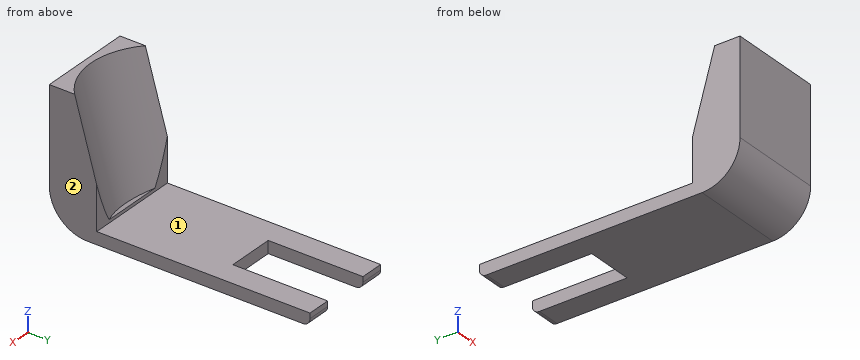
```python
from build123d import *

# Parameters (mm, degrees)
BOX001_W            = 10
BOX001_H            = 25
BOX001_DEPTH        = 10
BOX_W               = 20
BOX_H               = 45
BOX_DEPTH           = 2.6
CYLINDER_R          = 15
CYLINDER_DEPTH      = 27
CYLINDER_ROLL_ANGLE = 15.99999
BOX002_W            = 20
BOX002_H            = 10
BOX002_DEPTH        = 28
FILLET_R            = 8
FILLET001_R         = 1.5


with BuildPart() as box02:
    # Box001 → Box001 (new body)
    with BuildSketch(Plane(origin=(5, 25, -3), x_dir=(1, 0, 0), z_dir=(0, 0, 1))):
        with Locations((5, 12.5)):
            Rectangle(BOX001_W, BOX001_H)
    extrude(amount=BOX001_DEPTH)


with BuildPart() as obj1:
    # Box → Box (new body)
    with BuildSketch(Plane.XY):
        with Locations((10, 22.5)):
            Rectangle(BOX_W, BOX_H)
    extrude(amount=BOX_DEPTH)

    # Cut: cut Box02
    add(box02.part, mode=Mode.SUBTRACT)


with BuildPart() as cylinder:
    # Cylinder → Cylinder (new body)
    with BuildSketch(Plane.XY):
        Circle(CYLINDER_R)
    extrude(amount=CYLINDER_DEPTH)


with BuildPart() as cylinder_1:
    # Cylinder roll: moved
    add(cylinder.part.rotate(Axis((0, 0, 0), (1, 0, 0)), CYLINDER_ROLL_ANGLE))


with BuildPart() as cylinder_2:
    # Cylinder placement: moved
    add(cylinder_1.part.moved(Location((10, 13, 7))))


with BuildPart() as fillet001:
    # Box002 → Box002 (new body)
    with BuildSketch(Plane(origin=(0, -10, 0), x_dir=(1, 0, 0), z_dir=(0, 0, 1))):
        with Locations((10, 5)):
            Rectangle(BOX002_W, BOX002_H)
    extrude(amount=BOX002_DEPTH)

    # Fillet
    fillet_edges = [fillet001.edges().sort_by_distance(p)[0] for p in [
        (10, -10, 0),
    ]]
    fillet(fillet_edges, radius=FILLET_R)

    # Cut001: cut Cylinder
    add(cylinder_2.part, mode=Mode.SUBTRACT)

    # Fusion: union obj1
    add(obj1.part)

    # Fillet001
    fillet001_edges = [fillet001.edges().sort_by_distance(p)[0] for p in [
        (17.5, 45, 0),
        (2.5, 45, 0),
    ]]
    fillet(fillet001_edges, radius=FILLET001_R)


solid = fillet001.part
```
For this review, take the finished solid that the model builds, in its own axes (mm). Face numbers are marked on the shaded views. A direction names the side the tool comes from. Coordinates: 2 decimals unless noted, no trailing zeros. Order: outer loops, then holes, each group sorted by start corner. A loop starts at its lowest first (then second) coordinate and runs counter-clockwise, first axis right, second up. Notation, with made-up numbers: (41.25, 71.5) -> (46.25, 71.5) arc R14 ccw to (46.25, 88.5) -> close; hole circle Ø7 at (86.25, 3.5). An arc over 180 degrees is marked (long way). Use CSV: the item, a comma, the result in double quotes. Start each with the question number.
Item 1: We need section C-C, the plane y = 7.5. Give the boundary of the cut face in (x, z), then the cut area to 3 significant figures.
Item 2: Insertion check: pin 1 (3 mm diameter, centred on x = 6, z = 6.5, fed in from +Y); pin 2 (0.8 mm diameter, centred on x = 10.5, z = 1, fed in from +Y); pin 3 (5 mm diameter, centred on x = 18, z = 11.5, fed in from +Y). Each pin has a flat end and moves straight along its axis. Give the tip position at first contact, or say it passes through.
Item 3: We need section A-A, the plane y = 39. Give the boundary of the cut face in (x, z), then the cut area to 3 significant figures.
Item 4: We need section D-D, the plane x = 6.25. Give the boundary of the cut face in (y, z), then the cut area to 3 significant figures.
Item 5: Wall thickness on probe 1 along Z at (x, y) = (5.5, 9); probe 2 along Y at (x, z) = (18.25, 6); probe 3 along Y at (x, z) = (16.5, 19.75): over which ranges is each line inside the solid? List them lowest first.
Item 6: For the marked faces 1 and 2, list the 3-axis set-ups (+Z, -Z, +X, -X, +Y, -Y) from which the entire face can be reached by the end or side of a thin tool; tool diameter is ignored.
Item 7: We need section B-B, the plane x = 2. Give the boundary of the cut face in (y, z), then the cut area to 3 significant figures.
Derived:
1,outline,"(0, 0) -> (20, 0) -> (20, 2.6) -> (0, 2.6) -> close"
1,area,"52.0 mm^2"
2,pin 1,"stops at y = -1.24"
2,pin 2,"stops at y = 25"
2,pin 3,"stops at y = 0"
3,outline,"(0, 0) -> (5, 0) -> (5, 2.6) -> (0, 2.6) -> close; (15, 0) -> (20, 0) -> (20, 2.6) -> (15, 2.6) -> close"
3,area,"26.0 mm^2"
4,outline,"(-10, 8) arc R8 ccw to (-2, 0) -> (25, 0) -> (25, 2.6) -> (0, 2.6) -> (0, 3.27) -> (-0.96, 3) -> (-8.13, 28) -> (-10, 28) -> close"
4,area,"218 mm^2"
5,probe 1,"z = 0 to 2.6"
5,probe 2,"y = -9.75 to 0"
5,probe 3,"y = -10 to -4.72"
6,face 1,"+Z, +X, -X, +Y"
6,face 2,"+Z, -Z, +X, +Y, -Y"
7,outline,"(-10, 8) arc R8 ccw to (-2, 0) -> (43.5, 0) arc R1.5 ccw to (45, 1.5) -> (45, 2.6) -> (0, 2.6) -> (0, 6.3) -> (-6.22, 28) -> (-10, 28) -> close"
7,area,"315 mm^2"
